Print and shaded views of the part. All mm, measured from the part's lowest x, y and z. Round coordinates to 2 decimals unless told otherwise and drop trailing zeros. Loops run counter-clockwise (first coordinate to the right, second up) from the corner with the lowest first, then second, coordinate; pieces in that order, holes last. Notation, with made-up numbers: (8, 8) - (52, 8) arc R17 cw to (52, 36) - close; hole circle Ø2 at (45, 41). An arc over 180 degrees is marked (long way). Answer as a JSON object with one key per item and string values.
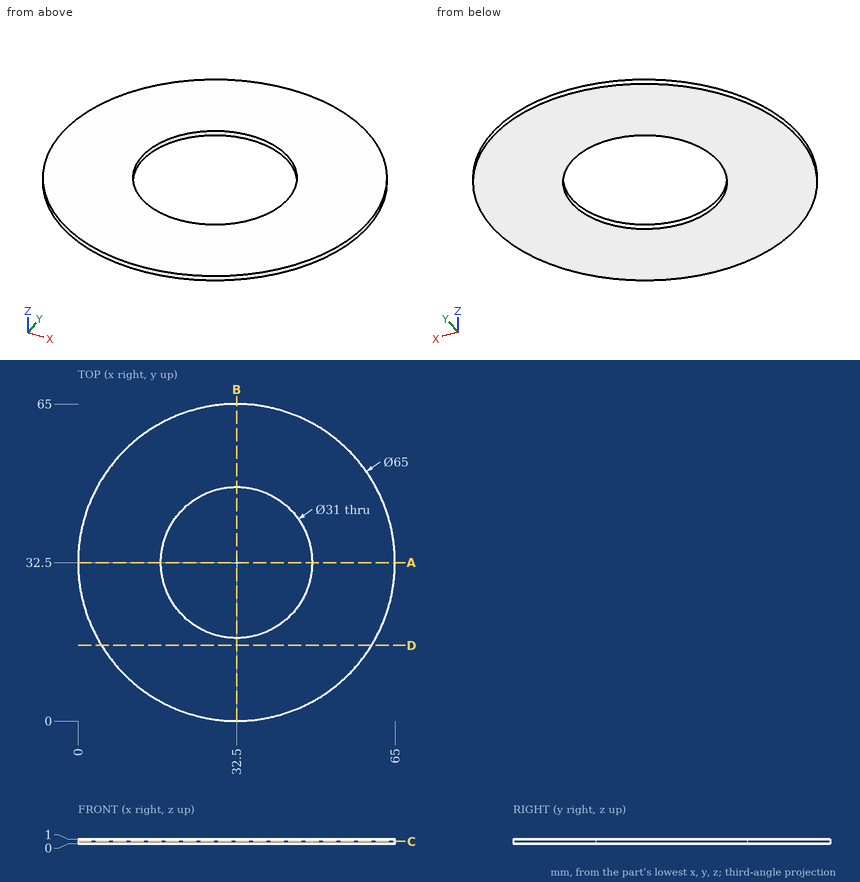
1) Drop a flat-ended pin along its axis: P1, Ø6, axis at x = 33, y = 22.5, coming from the +Z side. Give the stop position or say it passes through.
Values follow:
{"P1": "through"}
2) Slice it at C-C on z = 0.5. List the corners of the cut face in (x, y), then the cut area to 3 significant figures.
Values follow:
{"outline": "circle Ø65 at (32.5, 32.5); hole circle Ø31 at (32.5, 32.5)", "area": "2,560 mm²"}
3) Slice it at A-A on y = 32.5. List the corners of the cut face in (x, z).
Values follow:
{"outline": "(0, 0) - (17, 0) - (17, 1) - (0, 1) - close; (48, 0) - (65, 0) - (65, 1) - (48, 1) - close"}
4) Slice it at D-D on y = 15.5. List the corners of the cut face in (x, z).
Values follow:
{"outline": "(4.8, 0) - (60.2, 0) - (60.2, 1) - (4.8, 1) - close"}
5) Probe probe 1 along Y at (x, z) = (32.5, 0.4); probe 2 along X at (y, z) = (27, 0.8); probe 3 along X at (y, z) = (40.5, 0.85). List the from-to ranges inside material, lowest first.
Values follow:
{"probe 1": "0 to 17, 48 to 65", "probe 2": "0.47 to 18.01, 46.99 to 64.53", "probe 3": "1 to 19.22, 45.78 to 64"}
